```python
from build123d import *

# Parameters (mm, degrees)
SKETCH1_R           = 20
SKETCH1_R_2         = 17
BOSS_EXTRUDE1_DEPTH = 20
SKETCH2_R           = 20
BOSS_EXTRUDE2_DEPTH = 2
FILLET1_R           = 2


with BuildPart() as part:
    # Sketch1 → Boss-Extrude1 (new body)
    with BuildSketch(Plane.XY):
        Circle(SKETCH1_R)
        Circle(SKETCH1_R_2, mode=Mode.SUBTRACT)
    extrude(amount=BOSS_EXTRUDE1_DEPTH)

    # Sketch2 → Boss-Extrude2 (add)
    with BuildSketch(Plane.XY.offset(20)):
        Circle(SKETCH2_R)
    extrude(amount=BOSS_EXTRUDE2_DEPTH)

    # Fillet1
    fillet1_edges = [part.edges().sort_by_distance(p)[0] for p in [
        (-20, 0, 22),
    ]]
    fillet(fillet1_edges, radius=FILLET1_R)


solid = part.part
```
Source: CAD feature listing. Evaluate the final solid. Frame: model axes, mm. A direction names the side the tool comes from. Round coordinates to 2 decimals unless told otherwise and drop trailing zeros. Order: outer loops, then holes, each group sorted by start corner. A loop starts at its lowest first (then second) coordinate and runs counter-clockwise, first axis right, second up. Notation, with made-up numbers: (50.5, 18.5) -> (105.5, 18.5) arc R16 cw to (105.5, 32.5) -> close; hole circle Ø10 at (48.25, 39). An arc over 180 degrees is marked (long way). Use CSV: the item, a comma, the result in double quotes.
(1) Section A-A on x = 0. Return the cut outline in (y, z), and give its area (3 significant figures).
Report:
outline,"(-20, 0) -> (-17, 0) -> (-17, 20) -> (17, 20) -> (17, 0) -> (20, 0) -> (20, 20) arc R2 ccw to (18, 22) -> (-18, 22) arc R2 ccw to (-20, 20) -> close"
area,"198 mm^2"
(2) First-contact query: pin 1 Ø10 at (x, z) = (8.5, 9) entering from -Y; pin 2 Ø4 at (y, z) = (-12, 3) entering from +X; pin 3 Ø6 at (y, z) = (13, 5) entering from -X; pin 4 Ø6 at (y, z) = (-0.5, 5.5) entering from +X. Flat tips, straight axial feed; report the tip coordinate or a pass-through.
Report:
pin 1,"y = -19.69"
pin 2,"x = 17.32"
pin 3,"x = -17.32"
pin 4,"x = 20"
(3) Pull-direction query (Y, two-part tool) for faces 3 (the face through (-4.336, -19.524, 9.86)), 4 (the face through (0, 0, 20)), 5 (the face through (-9, -15, 0)); classes: +Y half, -Y half, draft (parallel to the pull), parting line (faces both ways), or undercut.
Report:
face 3,"parting line"
face 4,"undercut"
face 5,"draft"
(4) Access query for faces 1 (the face through (0, 0, 22)), 2 (the face through (9.139, 14.334, 9.86)). Directions: +Z, -Z, +X, -X, +Y, -Y. A direction counts if a zero-diameter tool reaches every point of the face in a straight line with its end or side. Return the directions, or none.
Report:
face 1,"+Z, +X, -X, +Y, -Y"
face 2,"-Z"
(5) Section B-B on z = 5. Return the cut outline in (x, y).
Report:
outline,"circle Ø40 at (0, 0); hole circle Ø34 at (0, 0)"
(6) Ray query, L1, parallel to Y at x = 0, z = 4.5; L2, parallel to Z at x = -10, y = 10; L3, parallel to X at y = -13, z = 19.75. Return the intervals inside material, ascending.
Report:
L1,"-20 to -17, 17 to 20"
L2,"20 to 22"
L3,"-15.2 to -10.95, 10.95 to 15.2"
